Design review of the part built by this model. Coordinates are the model's own, in mm. A direction names the side the tool comes from. Give positions to 0.01 mm unless a question says otherwise; leave off trailing zeros. Write each loop counter-clockwise with the first axis right and the second up, starting at its lowest first coordinate (ties: lowest second). Pieces come first, ordered by that corner, then holes. Notation, with made-up numbers: (30, -37.5) -> (57, -37.5) arc R29 ccw to (57, -15.5) -> close; hole circle Ø1 at (-2, 1.25). An arc over 180 degrees is marked (long way). Write each question's results on one line, items separated by ' | '. Start each with the question number.
(1) For faces 4 (the face through (593, -698.138, 401)), 5 (the face through (1270.517, -702, 401)), 6 (the face through (766, 38.462, 401)), list the 3-axis set-ups (+Z, -Z, +X, -X, +Y, -Y) from which the entire face can be reached by the end or side of a thin tool; tool diameter is ignored.
(2) Take a section at D-D (z = 62). State the section outline as (x, y) points, plus the area to 3 significant figures.
(3) Clearance check with flat-ended pins moving along their axes: pin 1 (8 mm diameter, centred on y = -720.5, z = 652.5, fed in from +X); pin 2 (6 mm diameter, centred on x = 1324, z = 433.5, fed in from -Y). State where each tip first meets the part, or that it passes through.
(4) Mouldability with a two-part tool opening along Z and no side actions: class faces 1 (the face through (1682.606, -251.495, 337.735)), 2 (the face through (465.356, -839.794, 577.739)), 3 (the face through (1010, -462, 812.8)) as released by +Z, released by -Z, zero draft, split by the parting line, or undercut.
(5) Take a section at B-B (y = -727.5). State the section outline as (x, z) points.
(6) Take a section at C-C (x = 1529.5). State the section outline as (y, z) points, plus the area to 3 significant figures.
(7) To check wall thickness, follow probe 1 along Y at (x, z) = (900.5, 125.5); probe 2 along X at (y, z) = (-774, 406); probe 3 along X at (y, z) = (-596.5, 630). State the ranges of each line that lie inside material, in increasing order.
(8) Take a section at A-A (z = 316). State the section outline as (x, y) points, plus the area to 3 significant figures.
from build123d import *

# Parameters (mm, degrees)
F1_DEPTH = 812.8
F3_DEPTH = 1016.001
F4_W     = 812.8
F4_H     = 457.2
F5_DEPTH = 812.8
F7_DEPTH = 812.8
F8_R     = 203.2
F9_DEPTH = 1016.001


with BuildPart() as f1:
    # F0 (on Top) → F1 (new body)
    with BuildSketch(Plane.XY):
        Polygon((1270.516747, 38.461771), (-50.283253, 38.461771), (-50.283253, -240.938229), (991.116747, -240.938229), (991.116747, -698.138229), (-50.283253, -698.138229), (-50.283253, -977.538229), (1270.516747, -977.538229), align=None)
    extrude(amount=F1_DEPTH)

    # F2 (on face) → F3 (cut, through all)
    with BuildSketch(Plane(origin=(0, 38.461771, 0), x_dir=(-1, 0, 0), z_dir=(0, 1, 0))):
        with BuildLine():
            Line((50.283253, 406.4), (50.283253, 812.8))
            Line((50.283253, 812.8), (-356.116747, 812.8))
            ThreePointArc((-356.116747, 812.8), (-68.748551, 693.768196), (50.283253, 406.4))
        make_face()
        with BuildLine():
            Line((50.283253, 0), (50.283253, 406.4))
            ThreePointArc((50.283253, 406.4), (-68.748551, 119.031804), (-356.116747, 0))
            Line((-356.116747, 0), (50.283253, 0))
        make_face()
    extrude(amount=-F3_DEPTH, mode=Mode.SUBTRACT)

    # F4 (on face) → F5 (join)
    with BuildSketch(Plane.XY.offset(812.8)):
        with Locations((1676.916747, -469.538229)):
            Rectangle(F4_W, F4_H)
    extrude(amount=-F5_DEPTH)

    # F6 (on face) → F7 (cut)
    with BuildSketch(Plane.YZ.offset(2083.316747)):
        with BuildLine():
            ThreePointArc((-698.138229, 406.4), (-469.538229, 635), (-240.938229, 406.4))
            Line((-240.938229, 406.4), (-240.938229, 812.8))
            Line((-240.938229, 812.8), (-698.138229, 812.8))
            Line((-698.138229, 812.8), (-698.138229, 406.4))
        make_face()
        with BuildLine():
            Line((-240.938229, 0), (-240.938229, 406.4))
            ThreePointArc((-240.938229, 406.4), (-469.538229, 177.8), (-698.138229, 406.4))
            Line((-698.138229, 406.4), (-698.138229, 0))
            Line((-698.138229, 0), (-240.938229, 0))
        make_face()
    extrude(amount=-F7_DEPTH, mode=Mode.SUBTRACT)

    # F8 (on face) → F9 (cut, through all)
    with BuildSketch(Plane.XZ.offset(977.538229)):
        with Locations((356.116747, 406.4)):
            Circle(F8_R)
    extrude(amount=-F9_DEPTH, mode=Mode.SUBTRACT)


solid = f1.part
Report:
1) face 4: +Z, -Z, -X | face 5: +X | face 6: +Z, -Z, +X, -X, +Y
2) outline: (140.36, -977.54) -> (1270.52, -977.54) -> (1270.52, 38.46) -> (140.36, 38.46) -> (140.36, -240.94) -> (991.12, -240.94) -> (991.12, -698.14) -> (140.36, -698.14) -> close | area: 759,000 mm2
3) pin 1: x = 1270.52 | pin 2: y = -696.86
4) face 1: split by the parting line | face 2: undercut | face 3: released by +Z
5) outline: (356.12, 0) -> (1270.52, 0) -> (1270.52, 812.8) -> (356.12, 812.8) arc R406.4 ccw to start; hole circle Ø406.4 at (356.12, 406.4)
6) outline: circle Ø457.2 at (-469.54, 406.4) | area: 164,000 mm2
7) probe 1: -977.54 to -698.14, -240.94 to 38.46 | probe 2: -50.28 to 152.92, 559.32 to 1270.52 | probe 3: 991.12 to 1270.52
8) outline: (-40.1, -977.54) -> (174.13, -977.54) -> (174.13, -698.14) -> (-40.1, -698.14) -> close; (-40.1, -240.94) -> (174.13, -240.94) -> (174.13, 38.46) -> (-40.1, 38.46) -> close; (538.1, -977.54) -> (1270.52, -977.54) -> (1270.52, -679.5) -> (2083.32, -679.5) -> (2083.32, -259.57) -> (1270.52, -259.57) -> (1270.52, 38.46) -> (538.1, 38.46) -> (538.1, -240.94) -> (991.12, -240.94) -> (991.12, -698.14) -> (538.1, -698.14) -> close | area: 998,000 mm2
